```python
from build123d import *

# Parameters (mm, degrees)
SKETCH1_R           = 1.5
SKETCH1_R_2         = 55
BOSS_EXTRUDE1_DEPTH = 3.175
CUT_EXTRUDE3_DEPTH  = 140.736059076
CUT_EXTRUDE4_DEPTH  = 140.736059076
CUT_EXTRUDE5_DEPTH  = 140.736059076
SKETCH6_R           = 1.5
CUT_EXTRUDE6_DEPTH  = 130.738840902
CUT_EXTRUDE7_DEPTH  = 10


with BuildPart() as part:
    # Sketch1 → Boss-Extrude1 (new body)
    with BuildSketch(Plane(origin=(0, 0, 0), x_dir=(1, 0, 0), z_dir=(0, 1, 0))):
        Polygon((0.047005036, -98.782806148), (-98.782806148, -0.047005036), (-0.047005036, 98.782806148), (98.782806148, 0.047005036), align=None)
        with Locations(Location((-61.346730494, 5.55625, 0), (0, 0, 270))):
            Circle(SKETCH1_R, mode=Mode.SUBTRACT)
        with Locations(Location((-61.346730494, -5.55625, 0), (0, 0, 270))):
            Circle(SKETCH1_R, mode=Mode.SUBTRACT)
        with Locations(Location((-5.55625, -61.346730494, 0), (0, 0, 270))):
            Circle(SKETCH1_R, mode=Mode.SUBTRACT)
        with Locations(Location((5.55625, -61.346730494, 0), (0, 0, 270))):
            Circle(SKETCH1_R, mode=Mode.SUBTRACT)
        with Locations(Location((61.346730494, -5.55625, 0), (0, 0, 270))):
            Circle(SKETCH1_R, mode=Mode.SUBTRACT)
        with Locations(Location((61.346730494, 5.55625, 0), (0, 0, 270))):
            Circle(SKETCH1_R, mode=Mode.SUBTRACT)
        with Locations(Location((5.55625, 61.346730494, 0), (0, 0, 270))):
            Circle(SKETCH1_R, mode=Mode.SUBTRACT)
        with Locations(Location((-5.55625, 61.346730494, 0), (0, 0, 270))):
            Circle(SKETCH1_R, mode=Mode.SUBTRACT)
        with Locations(Location((0, 0, 0), (0, 0, 270))):
            Circle(SKETCH1_R_2, mode=Mode.SUBTRACT)
    extrude(amount=BOSS_EXTRUDE1_DEPTH)

    # Sketch2 → Cut-Extrude3 (cut, through all)
    with BuildSketch(Plane(origin=(0, 3.175, 0), x_dir=(1, 0, 0), z_dir=(0, 1, 0))):
        Polygon((3.175, 53.34), (3.175, 59.69), (-3.175, 59.69), (-3.175, 53.34), (-3.175, 52.244537665), (3.175, 52.244537665), align=None)
        Polygon((53.34, -3.175), (59.69, -3.175), (59.69, 3.175), (53.34, 3.175), (52.244537665, 3.175), (52.244537665, -3.175), align=None)
        Polygon((-3.175, -53.34), (-3.175, -59.69), (3.175, -59.69), (3.175, -53.34), (3.175, -52.244537665), (-3.175, -52.244537665), align=None)
        Polygon((-53.34, 3.175), (-59.69, 3.175), (-59.69, -3.175), (-53.34, -3.175), (-52.244537665, -3.175), (-52.244537665, 3.175), align=None)
    extrude(amount=-CUT_EXTRUDE3_DEPTH, mode=Mode.SUBTRACT)

    # Sketch3 → Cut-Extrude4 (cut, through all)
    with BuildSketch(Plane(origin=(0, 3.175, 0), x_dir=(1, 0, 0), z_dir=(0, 1, 0))):
        Polygon((-49.414905592, 49.367900556), (49.414905592, -49.367900556), (0.047005036, -98.782806148), (-98.782806148, -0.047005036), align=None)
    extrude(amount=-CUT_EXTRUDE4_DEPTH, mode=Mode.SUBTRACT)

    # Sketch5 → Cut-Extrude5 (cut, through all)
    with BuildSketch(Plane(origin=(0, 3.175, 0), x_dir=(1, 0, 0), z_dir=(0, 1, 0))):
        Polygon((98.782806148, 0.047005036), (91.71510385, -7.027426688), (-7.114707335, 91.708374424), (-0.047005036, 98.782806148), align=None)
    extrude(amount=-CUT_EXTRUDE5_DEPTH, mode=Mode.SUBTRACT)

    # Sketch6 → Cut-Extrude6 (cut, through all)
    with BuildSketch(Plane(origin=(0, 3.175, 0), x_dir=(1, 0, 0), z_dir=(0, 1, 0))):
        with Locations(Location((64.725061333, -22.363275374, 0), (0, 0, 270))):
            Circle(SKETCH6_R)
        with Locations(Location((75.300110897, -11.778156907, 0), (0, 0, 270))):
            Circle(SKETCH6_R)
        with Locations(Location((-12.20223816, 74.702563661, 0), (0, 0, 90))):
            Circle(SKETCH6_R)
        with Locations(Location((-22.662437607, 64.003936002, 0), (0, 0, 90))):
            Circle(SKETCH6_R)
        with Locations(Location((54.443600685, -33.241703487, 0), (0, 0, 270))):
            Circle(SKETCH6_R)
        with Locations(Location((-33.419374261, 53.595432504, 0), (0, 0, 90))):
            Circle(SKETCH6_R)
    extrude(amount=-CUT_EXTRUDE6_DEPTH, mode=Mode.SUBTRACT)

    # Sketch7 → Cut-Extrude7 (cut)
    with BuildSketch(Plane(origin=(0, 3.175, 0), x_dir=(1, 0, 0), z_dir=(0, 1, 0))):
        Polygon((49.414905592, -49.367900556), (57.268889772, -41.506438303), (-41.560921413, 57.229362809), (-49.414905592, 49.367900556), align=None)
    extrude(amount=-CUT_EXTRUDE7_DEPTH, mode=Mode.SUBTRACT)


solid = part.part
```
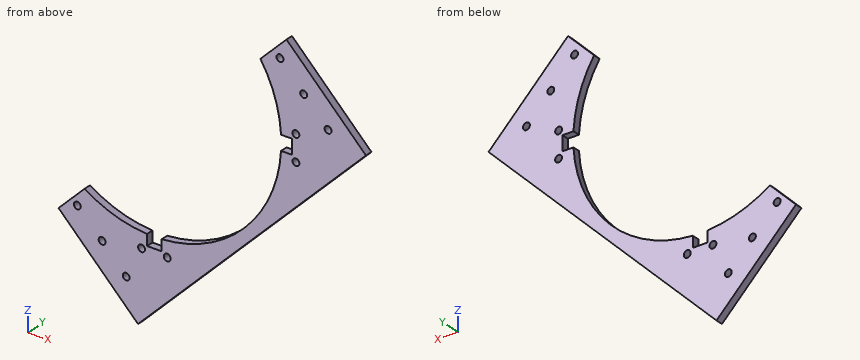
The model under review builds one solid part; all positions refer to its coordinate system, in mm. Round coordinates to 2 decimals unless told otherwise and drop trailing zeros. Loops run counter-clockwise (first coordinate to the right, second up) from the corner with the lowest first, then second, coordinate; pieces in that order, holes last.
Item 1: Take a section at B-B (z = 27). Write out the cut boundary in (x, y) (3 decimals), then the cut area to 3 significant figures.
Determined:
outline: (47.917, 0) - (71.762, 0) - (71.762, 3.175) - (47.917, 3.175) - close
area: 75.7 mm2
Item 2: For line 1 (X direction, y = 0.2, z = -5); line 2 (Z direction, x = 47, y = 0.95); line 3 (X direction, y = 2.05, z = 12.5) (3 decimals), list the stretches that pass through material, from the lowest coordinate up.
Determined:
line 1: x = 54.77 to 59.95, 62.74 to 79.68
line 2: z = -37.65 to -28.57, 28.57 to 31.25
line 3: x = 53.561 to 73.985, 76.615 to 86.248
Item 3: Clearance check with flat-ended pins moving along their axes: pin 1 Ø1 at (y, z) = (2, -14.5) entering from +X; pin 2 Ø1.6 at (y, z) = (2, -56.5) entering from +X; pin 3 Ø1 at (x, y) = (58, 2) entering from +Z. State where each tip first meets the part, or that it passes through.
Determined:
pin 1: stops at x = 70.67
pin 2: stops at x = 28.93
pin 3: stops at z = 41.28
Item 4: Take a section at C-C (x = 12). Write out the cut boundary in (y, z) (3 decimals), then the cut area to 3 significant figures.
Determined:
outline: (0, -72.612) - (3.175, -72.612) - (3.175, -53.675) - (0, -53.675) - close
area: 60.1 mm2
Item 5: Take a section at A-A (y = 2.35). Give the number of separate pieces and of enclosed holes in the cut face, then the cut area to 3 significant figures.
Determined:
separate pieces: 1
enclosed holes: 10
area: 3,140 mm2
